from build123d import *

# Parameters (mm, degrees)
F0_W     = 76.2
F0_H     = 58.42
F0_W_2   = 71.12
F0_H_2   = 53.34
F1_DEPTH = 50.8
F2_W     = 50.8
F2_H     = 7.62
F6_DEPTH = 22.86
F7_W     = 50.8
F7_H     = 7.62
F8_DEPTH = 35.56
F3_W     = 20.32
F3_H     = 48.26
F9_DEPTH = 2.54
F4_W     = 22.86
F4_H     = 33.02
F5_DEPTH = 2.54


with BuildPart() as f1:
    # F0 (on Top) → F1 (new body)
    with BuildSketch(Plane.XY):
        with Locations((31.363072, -14.94423)):
            Rectangle(F0_W, F0_H)
        with Locations((31.363072, -14.94423)):
            Rectangle(F0_W_2, F0_H_2, mode=Mode.SUBTRACT)
    extrude(amount=F1_DEPTH)

    # F2 (on face) → F6 (join)
    with BuildSketch(Plane.XZ.offset(-11.72577)):
        with Locations((41.523072, 24.13)):
            Rectangle(F2_W, F2_H)
    extrude(amount=F6_DEPTH)

    # F7 (on face) → F8 (join)
    with BuildSketch(Plane(origin=(66.923072, 0, 0), x_dir=(0, -1, 0), z_dir=(-1, 0, 0))):
        with Locations((13.67423, 3.81)):
            Rectangle(F7_W, F7_H)
    extrude(amount=F8_DEPTH)

    # F3 (on face) → F9 (cut, through all)
    with BuildSketch(Plane(origin=(-6.736928, 0, 0), x_dir=(0, -1, 0), z_dir=(-1, 0, 0))):
        with Locations((14.370841, 24.13)):
            Rectangle(F3_W, F3_H)
    extrude(amount=-F9_DEPTH, mode=Mode.SUBTRACT)

    # F4 (on face) → F5 (cut, through all)
    with BuildSketch(Plane.XZ.offset(44.15423)):
        with Locations((44.301499, 27.94)):
            Rectangle(F4_W, F4_H)
    extrude(amount=-F5_DEPTH, mode=Mode.SUBTRACT)


solid = f1.part
Can you work these out from the model? Positions are in its coordinate system, mm. A direction names the side the tool comes from. Give positions to 0.01 mm unless a question says otherwise; leave off trailing zeros. Order: outer loops, then holes, each group sorted by start corner. A loop starts at its lowest first (then second) coordinate and runs counter-clockwise, first axis right, second up. Notation, with made-up numbers: M 87.5,82 L 107.5,82 A32 cw 107.5,110 Z; hole C 79.25,28 d9. An arc over 180 degrees is marked long. Use a Markdown table: item, result. Add a question column.
Item 1: Suppose I cut it at D-D (x = 41.5). List the corners of the cut face in (y, z) for me.
Item 2: If I drill on L1, parallel to Y at x = 16, z = 29; L2, parallel to X at y = -27.5, z = 42.5; L3, parallel to Z at x = 33, y = -7, over which ranges is the centre line in solid material (lowest first)? Write a range as [from, to].
Item 3: We'd pull the mould along Y, two halves only. Please class faces 4 (the flat face through (31, 14.266, 25)), 5 (the flat face through (28, -43, 50.8)), 6 (the flat face through (41, 0, 20.32)): +Y half, -Y half, draft (parallel to the pull), parting line (faces both ways), or undercut.
Item 4: For faces 1 (the flat face through (66.923, -15, 31)), 2 (the flat face through (-5, -14, 48.26)), 3 (the flat face through (31.363, -13, 4)), which set-ups out of +Z, -Z, +X, -X, +Y, -Y let a thin tool reach every point of the face, with its end or its side?
Item 5: Suppose I cut it at A-A (y = 6). List the corners of the cut face in (x, z) for me.
Item 6: Will these pins go through, and if not, where does the flat tip stop? pin 1 (11.5 mm diameter, centred on x = 48.5, y = 1.5, fed in from -Z); pin 2 (18 mm diameter, centred on x = 50.5, y = -19.5, fed in from +Z); pin 3 (1.5 mm diameter, centred on y = -13, z = 13.5, fed in from -X); pin 4 (3 mm diameter, centred on x = -5.5, y = -18, fed in from -Z).
Item 7: Suppose I cut it at C-C (z = 26.5). List the corners of the cut face in (x, y) for me, then the cut area to 3 significant figures.
Item 8: Suppose I cut it at B-B (x = -0.5). List the corners of the cut face in (y, z) for me.
Answer sheet:
| question | item | result |
|---|---|---|
| 1 | outline | M -44.15,0 L -41.61,0 L -41.61,11.43 L -44.15,11.43 Z; M -44.15,44.45 L -41.61,44.45 L -41.61,50.8 L -44.15,50.8 Z; M -39.07,0 L 14.27,0 L 14.27,50.8 L 11.73,50.8 L 11.73,27.94 L -11.13,27.94 L -11.13,20.32 L 11.73,20.32 L 11.73,7.62 L -39.07,7.62 Z |
| 2 | L1 | y = [-44.15, -41.61], [11.73, 14.27] |
| 2 | L2 | x = [-6.74, -4.2], [66.92, 69.46] |
| 2 | L3 | z = [0, 7.62], [20.32, 27.94] |
| 3 | face 4 | +Y half |
| 3 | face 5 | draft |
| 3 | face 6 | undercut |
| 4 | face 1 | none |
| 4 | face 2 | -Z, -X |
| 4 | face 3 | -Z |
| 5 | outline | M -6.74,0 L -4.2,0 L -4.2,50.8 L -6.74,50.8 Z; M 16.12,20.32 L 66.92,20.32 L 66.92,7.62 L 31.36,7.62 L 31.36,0 L 69.46,0 L 69.46,50.8 L 66.92,50.8 L 66.92,27.94 L 16.12,27.94 Z |
| 6 | pin 1 | stops at z = 0 |
| 6 | pin 2 | stops at z = 27.94 |
| 6 | pin 3 | stops at x = 66.92 |
| 6 | pin 4 | stops at z = 48.26 |
| 7 | outline | M -6.74,-44.15 L 32.87,-44.15 L 32.87,-41.61 L -4.2,-41.61 L -4.2,-24.53 L -6.74,-24.53 Z; M -6.74,-4.21 L -4.2,-4.21 L -4.2,11.73 L 16.12,11.73 L 16.12,-11.13 L 66.92,-11.13 L 66.92,-41.61 L 55.73,-41.61 L 55.73,-44.15 L 69.46,-44.15 L 69.46,14.27 L -6.74,14.27 Z |
| 7 | area | 1,710 mm² |
| 8 | outline | M -44.15,0 L -41.61,0 L -41.61,50.8 L -44.15,50.8 Z; M 11.73,0 L 14.27,0 L 14.27,50.8 L 11.73,50.8 Z |
